```python
from build123d import *

# Parameters (mm, degrees)
F1_DEPTH = 30
F2_R     = 8
F3_DEPTH = 200
F5_R     = 2
F6_R     = 6
F4_R     = 5.25
F7_DEPTH = 25


# Not quite as in the source:
# - a feature names something its author has since deleted; it is built from what else it names


with BuildPart() as f1:
    # F0 (on Right) → F1 (new body, symmetric)
    with BuildSketch(Plane.YZ):
        Polygon((36, -50), (-40, -50), (-40, 46), (-44, 46), (-44, -54), (36, -54), align=None)
    extrude(amount=F1_DEPTH, both=True)

    # F2 (on face) → F3 (join)
    with BuildSketch(Plane(origin=(0, 0, -54), x_dir=(1, 0, 0), z_dir=(0, 0, -1))):
        Circle(F2_R)
    extrude(amount=F3_DEPTH)

    # F5
    f5_edges = [f1.edges().sort_by_distance(p)[0] for p in [
        (0, -40, -50),
    ]]
    fillet(f5_edges, radius=F5_R)

    # F6
    f6_edges = [f1.edges().sort_by_distance(p)[0] for p in [
        (0, -44, -54),
    ]]
    fillet(f6_edges, radius=F6_R)

    # F4 (on face) → F7 (cut)
    with BuildSketch(Plane.XZ.offset(44)):
        with Locations((18, 34)):
            Circle(F4_R)
        with Locations((0, 5)):
            Circle(F4_R)
        with Locations((-18, -24)):
            Circle(F4_R)
    extrude(amount=-F7_DEPTH, mode=Mode.SUBTRACT)


solid = f1.part
```
Can you work these out from the model? Positions are in its coordinate system, mm. A direction names the side the tool comes from. Coordinates: 2 decimals unless noted, no trailing zeros. Write each loop counter-clockwise with the first axis right and the second up, starting at its lowest first coordinate (ties: lowest second). Pieces come first, ordered by that corner, then holes. Notation, with made-up numbers: M -25,-21.5 L 32,-21.5 A21 ccw 32,-5.5 Z; hole C 82.5,-27 d4. An arc over 180 degrees is marked long. Write item = value, one per line. Start each with the question number.
Q1. Thinking about a two-plate mould opening in X: for faces 1 (the face through (-30, -43, -26)), 2 (the face through (-6, -44, 0)), 3 (the face through (5, -42, 6.6)), which applies, released by +X, released by -X, zero draft, split by the parting line, or undercut?
Q2. If I drill on L1, parallel to Z at x = 13, y = -8.5; L2, parallel to X at y = -6, z = -141; L3, parallel to Y at x = 23.5, z = -32, over which ranges is the centre line in solid material (lowest first)? Write a range as [from, to].
Q3. On a 3-axis mill with a long thin cutter (end or side, diameter ignored), from which of +Z, -Z, +X, -X, +Y, -Y can I reach the whole of each face in a straight line? I mean faces 4 (the face through (0, -40, -2)), 5 (the face through (-1.73, 7.81, -152.6)), 6 (the face through (0, 0, -254)). Say none if no direction works.
Q4. If we section it at D-D, the plane x = -18: Write out the boundary of the cut face in (y, z).
Q5. If we section it at B-B, the plane z = 34: Write out the boundary of the cut face in (x, y).
Q6. I'm going to push flat-ended pins straight in: pin 1 (8.5 mm diameter, centred on x = 18, z = 34, fed in from +Y); pin 2 (3 mm diameter, centred on x = -1.5, z = -130, fed in from -Y); pin 3 (6 mm diameter, centred on x = -2.5, y = 13.5, fed in from -Z); pin 4 (3 mm diameter, centred on x = -2.5, z = -4, fed in from +Y). Where does each tip first touch, or does it pass through?
Q7. If we section it at A-A, the plane x = 0: Write out the boundary of the cut face in (y, z), then the cut area to 3 significant figures.
Q8. If we section it at C-C, the plane y = 0: Write out the boundary of the cut face in (x, z), then the cut area to 3 significant figures.
Check sheet entries:
q1.face_1 = released by -X
q1.face_2 = zero draft
q1.face_3 = undercut
q2.L1 = [-54, -50]
q2.L2 = [-5.29, 5.29]
q2.L3 = [-44, -40]
q3.face_4 = +Z, +X, -X, +Y
q3.face_5 = -Z
q3.face_6 = -Z, +X, -X, +Y, -Y
q4.outline = M -44,-48 A6 ccw -38,-54 L 36,-54 L 36,-50 L -38,-50 A2 cw -40,-48 L -40,-29.25 L -44,-29.25 Z; M -44,-18.75 L -40,-18.75 L -40,46 L -44,46 Z
q5.outline = M -30,-44 L 12.75,-44 L 12.75,-40 L -30,-40 Z; M 23.25,-44 L 30,-44 L 30,-40 L 23.25,-40 Z
q6.pin_1 = through
q6.pin_2 = -8
q6.pin_3 = -54
q6.pin_4 = -40
q7.outline = M -44,-48 A6 ccw -38,-54 L -8,-54 L -8,-254 L 8,-254 L 8,-54 L 36,-54 L 36,-50 L -38,-50 A2 cw -40,-48 L -40,-0.25 L -44,-0.25 Z; M -44,10.25 L -40,10.25 L -40,46 L -44,46 Z
q7.area = 3,860 mm²
q8.outline = M -30,-54 L -8,-54 L -8,-254 L 8,-254 L 8,-54 L 30,-54 L 30,-50 L -30,-50 Z
q8.area = 3,440 mm²
